Can you work these out from the model? Positions are in its coordinate system, mm. Face numbers are marked on the shaded views. A direction names the side the tool comes from. Round coordinates to 2 decimals unless told otherwise and drop trailing zeros. Loops run counter-clockwise (first coordinate to the right, second up) from the corner with the lowest first, then second, coordinate; pieces in that order, holes last. Notation, with made-up numbers: M 68,58.25 L 105,58.25 A25 ccw 105,77.25 Z; hole C -36.5,21.25 d10. An arc over 180 degrees is marked long. Answer as CSV lines item,"result".
from build123d import *

# Parameters (mm, degrees)
SKETCH1_R           = 3.4
BOSS_EXTRUDE1_DEPTH = 100
CUT_EXTRUDE1_DEPTH  = 101
CIRPATTERN1_COUNT   = 4


with BuildPart() as part:
    # Sketch1 → Boss-Extrude1 (new body)
    with BuildSketch(Plane(origin=(0, 0, 0), x_dir=(1, 0, 0), z_dir=(0, 1, 0))):
        with BuildLine():
            ThreePointArc((-15, -12.5), (-14.267766953, -14.267766953), (-12.5, -15))
            Line((-12.5, -15), (12.5, -15))
            ThreePointArc((12.5, -15), (14.267766953, -14.267766953), (15, -12.5))
            Line((15, -12.5), (15, 12.5))
            ThreePointArc((15, 12.5), (14.267766953, 14.267766953), (12.5, 15))
            Line((12.5, 15), (-12.5, 15))
            ThreePointArc((-12.5, 15), (-14.267766953, 14.267766953), (-15, 12.5))
            Line((-15, 12.5), (-15, -12.5))
        make_face()
        with BuildLine():
            Line((-12.672792206, -9.672792206), (-10.672792206, -9.672792206))
            ThreePointArc((-10.672792206, -9.672792206), (-9.965685425, -9.965685425), (-9.672792206, -10.672792206))
            Line((-9.672792206, -10.672792206), (-9.672792206, -12.672792206))
            ThreePointArc((-9.672792206, -12.672792206), (-9.965685425, -13.379898987), (-10.672792206, -13.672792206))
            Line((-10.672792206, -13.672792206), (-12.672792206, -13.672792206))
            ThreePointArc((-12.672792206, -13.672792206), (-13.379898987, -13.379898987), (-13.672792206, -12.672792206))
            Line((-13.672792206, -12.672792206), (-13.672792206, -10.672792206))
            ThreePointArc((-13.672792206, -10.672792206), (-13.379898987, -9.965685425), (-12.672792206, -9.672792206))
        make_face(mode=Mode.SUBTRACT)
        Polygon((-8.4, -9.672792206), (-4.427207794, -5.7), (4.427207794, -5.7), (8.4, -9.672792206), (8.4, -13.2), (-8.4, -13.2), align=None, mode=Mode.SUBTRACT)
        with BuildLine():
            Line((9.672792206, -12.672792206), (9.672792206, -10.672792206))
            ThreePointArc((9.672792206, -10.672792206), (9.965685425, -9.965685425), (10.672792206, -9.672792206))
            Line((10.672792206, -9.672792206), (12.672792206, -9.672792206))
            ThreePointArc((12.672792206, -9.672792206), (13.379898987, -9.965685425), (13.672792206, -10.672792206))
            Line((13.672792206, -10.672792206), (13.672792206, -12.672792206))
            ThreePointArc((13.672792206, -12.672792206), (13.379898987, -13.379898987), (12.672792206, -13.672792206))
            Line((12.672792206, -13.672792206), (10.672792206, -13.672792206))
            ThreePointArc((10.672792206, -13.672792206), (9.965685425, -13.379898987), (9.672792206, -12.672792206))
        make_face(mode=Mode.SUBTRACT)
        Polygon((-5.7, 4.427207794), (-5.7, -4.427207794), (-9.672792206, -8.4), (-13.2, -8.4), (-13.2, 8.4), (-9.672792206, 8.4), align=None, mode=Mode.SUBTRACT)
        with BuildLine():
            Line((-10.672792206, 9.672792206), (-12.672792206, 9.672792206))
            ThreePointArc((-12.672792206, 9.672792206), (-13.379898987, 9.965685425), (-13.672792206, 10.672792206))
            Line((-13.672792206, 10.672792206), (-13.672792206, 12.672792206))
            ThreePointArc((-13.672792206, 12.672792206), (-13.379898987, 13.379898987), (-12.672792206, 13.672792206))
            Line((-12.672792206, 13.672792206), (-10.672792206, 13.672792206))
            ThreePointArc((-10.672792206, 13.672792206), (-9.965685425, 13.379898987), (-9.672792206, 12.672792206))
            Line((-9.672792206, 12.672792206), (-9.672792206, 10.672792206))
            ThreePointArc((-9.672792206, 10.672792206), (-9.965685425, 9.965685425), (-10.672792206, 9.672792206))
        make_face(mode=Mode.SUBTRACT)
        Circle(SKETCH1_R, mode=Mode.SUBTRACT)
        Polygon((9.672792206, 8.4), (13.2, 8.4), (13.2, -8.4), (9.672792206, -8.4), (5.7, -4.427207794), (5.7, 4.427207794), align=None, mode=Mode.SUBTRACT)
        Polygon((4.427207794, 5.7), (-4.427207794, 5.7), (-8.4, 9.672792206), (-8.4, 13.2), (8.4, 13.2), (8.4, 9.672792206), align=None, mode=Mode.SUBTRACT)
        with BuildLine():
            Line((12.672792206, 9.672792206), (10.672792206, 9.672792206))
            ThreePointArc((10.672792206, 9.672792206), (9.965685425, 9.965685425), (9.672792206, 10.672792206))
            Line((9.672792206, 10.672792206), (9.672792206, 12.672792206))
            ThreePointArc((9.672792206, 12.672792206), (9.965685425, 13.379898987), (10.672792206, 13.672792206))
            Line((10.672792206, 13.672792206), (12.672792206, 13.672792206))
            ThreePointArc((12.672792206, 13.672792206), (13.379898987, 13.379898987), (13.672792206, 12.672792206))
            Line((13.672792206, 12.672792206), (13.672792206, 10.672792206))
            ThreePointArc((13.672792206, 10.672792206), (13.379898987, 9.965685425), (12.672792206, 9.672792206))
        make_face(mode=Mode.SUBTRACT)
    extrude(amount=BOSS_EXTRUDE1_DEPTH)

    # Sketch2 → Cut-Extrude1 (cut, through all)
    with BuildSketch(Plane(origin=(0, 100, 0), x_dir=(1, 0, 0), z_dir=(0, 1, 0))):
        Polygon((-4.1, 14.1), (-4.1, 13.2), (4.1, 13.2), (4.1, 14.1), (5.1, 14.1), (5.1, 15), (-5.1, 15), (-5.1, 14.1), align=None)
    cut_extrude1 = extrude(amount=-CUT_EXTRUDE1_DEPTH, mode=Mode.SUBTRACT)

    # CirPattern1: Cut-Extrude1 ×4 about axis
    cirpattern1_axis = Axis((0, 0, 0), (0, 1, 0))
    for i in range(1, CIRPATTERN1_COUNT):
        add(cut_extrude1.rotate(cirpattern1_axis, i * 360 / CIRPATTERN1_COUNT), mode=Mode.SUBTRACT)


solid = part.part
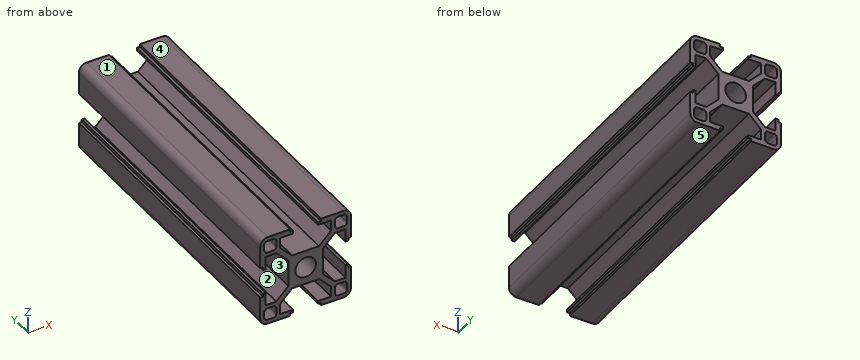
Item 1: If we section it at A-A on z = 0: Write out the boundary of the cut face in (x, y).
Output:
outline,"M -5.7,0 L -3.4,0 L -3.4,100 L -5.7,100 Z; M 3.4,0 L 5.7,0 L 5.7,100 L 3.4,100 Z"
Item 2: We'd pull the mould along Z, two halves only. Please class the marked faces 3, 4 and 5: released by +Z, released by -Z, zero draft, split by the parting line, or undercut.
Output:
face 3,"undercut"
face 4,"released by +Z"
face 5,"released by -Z"
Item 3: If I drill on line 1 along X through (y, z) = (50, 12); line 2 along Z through (x, y) = (-10.5, 20); line 3 along Z through (x, y) = (0, 12), over which ranges is the centre line in solid material (lowest first)? Write a range as from..to.
Output:
line 1,"x = -15..-13.67, -9.67..-8.4, 8.4..9.67, 13.67..15"
line 2,"z = -15..-13.66, -9.69..-8.4, 8.4..9.69, 13.66..15"
line 3,"z = -5.7..-3.4, 3.4..5.7"
Item 4: Will these pins go through, and if not, where does the flat tip stop? pin 1 (1 mm diameter, centred on y = 25.5, z = 14, fed in from +X); pin 2 (0.8 mm diameter, centred on y = 63, z = -4.5, fed in from +X); pin 3 (0.5 mm diameter, centred on y = 59, z = 13.5, fed in from -X).
Output:
pin 1,"stops at x = 14.79"
pin 2,"stops at x = 14.1"
pin 3,"stops at x = -14.88"
Item 5: If we section it at C-C on y = 32.5: State how many separate pieces and enclosed holes the cut face has, then the cut area to 3 significant figures.
Output:
separate pieces,"1"
enclosed holes,"5"
area,"291 mm2"
Item 6: On a 3-axis mill with a long thin cutter (end or side, diameter ignored), from which of +Z, -Z, +X, -X, +Y, -Y can I reach the whole of each face in a straight line? I mean the marked faces 1 and 2. Say none if no direction works.
Output:
face 1,"+Z, +X, -X, +Y, -Y"
face 2,"+Y, -Y"
Item 7: If we section it at B-B on x = 0: Write out the boundary of the cut face in (y, z).
Output:
outline,"M 0,-5.7 L 100,-5.7 L 100,-3.4 L 0,-3.4 Z; M 0,3.4 L 100,3.4 L 100,5.7 L 0,5.7 Z"
